from build123d import *

# Parameters (mm, degrees)
SKETCH_1_W             = 180
SKETCH_1_H             = 5
EXTRUDE_1_DEPTH        = 10
SKETCH_2_W             = 3
SKETCH_2_H             = 8
EXTRUDE_2_DEPTH        = 60
SKETCH_5_R             = 2
EXTRUDE_4_DEPTH        = 8
SKETCH_6_W             = 36
SKETCH_6_H             = 4
EXTRUDE_5_DEPTH        = 40
SKETCH_7_W             = 30
SKETCH_7_H             = 5
EXTRUDE_6_DEPTH        = 30
PATTERN_LINEAR_1_COUNT = 2
PATTERN_LINEAR_1_PITCH = 177.5
EXTRUDE_START          = 8
SKETCH_8_R             = 2
EXTRUDE_7_DEPTH        = 8


with BuildPart() as part:
    # 草图1 → 凸台-拉伸1 (new body)
    with BuildSketch(Plane(origin=(0, 0, 0), x_dir=(1, 0, 0), z_dir=(0, 1, 0))):
        Rectangle(SKETCH_1_W, SKETCH_1_H)
    extrude(amount=EXTRUDE_1_DEPTH)

    # 草图2 → 凸台-拉伸2 (add)
    with BuildSketch(Plane(origin=(0, 0, -2.5), x_dir=(-1, 0, 0), z_dir=(0, 0, -1))):
        with Locations((-88.5, 5)):
            Rectangle(SKETCH_2_W, SKETCH_2_H)
    extrude_2 = extrude(amount=EXTRUDE_2_DEPTH)

    # 草图5 → 凸台-拉伸4 (add)
    with BuildSketch(Plane.ZY.offset(-87)):
        with Locations(Location((-59.5, 5, 0), (0, 0, 180))):
            Circle(SKETCH_5_R)
    extrude(amount=EXTRUDE_4_DEPTH)

    # 草图6 → 凸台-拉伸5 (add)
    with BuildSketch(Plane.XY.offset(2.5)):
        with Locations((0, 5)):
            Rectangle(SKETCH_6_W, SKETCH_6_H)
    extrude(amount=EXTRUDE_5_DEPTH)

    # 草图7 → 凸台-拉伸6 (add)
    with BuildSketch(Plane.XZ.offset(-3)):
        with Locations((0, 40)):
            Rectangle(SKETCH_7_W, SKETCH_7_H)
    extrude(amount=EXTRUDE_6_DEPTH)

    # 阵列(线性)1: 凸台-拉伸2 ×2
    with Locations(*[(-i * PATTERN_LINEAR_1_PITCH, 0, 0) for i in range(1, PATTERN_LINEAR_1_COUNT)]):
        add(extrude_2)

    # 草图8 → 凸台-拉伸7 (add)
    with BuildSketch(Plane(origin=(-87.5, 0, 0), x_dir=(0, 0, -1), z_dir=(1, 0, 0)).offset(EXTRUDE_START)):
        with Locations((59.5, 5)):
            Circle(SKETCH_8_R)
    extrude(amount=-EXTRUDE_7_DEPTH)


solid = part.part
Geometry check sheet. Reference: the model listing, model coordinates, mm. A direction names the side the tool comes from. Round coordinates to 2 decimals unless told otherwise and drop trailing zeros. Loops run counter-clockwise (first coordinate to the right, second up) from the corner with the lowest first, then second, coordinate; pieces in that order, holes last.
Item 1: Mould release check, pull along X, two halves, no side actions. Record for faces 4 (the flat face through (79, 5, -59)), 5 (the flat face through (15, -12, 40)), 6 (the flat face through (-1, 0, 0)): pulls with the +X half, pulls with the -X half, needs draft (parallel to the pull), parting line crosses it, or undercut.
Item 2: Cross-section at B-B on y = 5. Record the boundary of the cut face in (x, z).
Item 3: Access from +Z, -Z, +X, -X, +Y, -Y to the whole of each face (thin tool, end or side, straight path). Record for faces 1 (the cylindrical face through (-83.444, 5.601, -61.408)), 2 (the flat face through (0, 7, 22)), 3 (the flat face through (-79.5, 5, -59)).
Item 4: Cross-section at A-A on z = -59.5. Record the boundary of the cut face in (x, y).
Item 5: Cross-section at C-C on x = 67. Record the boundary of the cut face in (y, z).
Item 6: Gauge pin test, flat ends, axial feed: pin 1 (9 mm diameter, centred on x = 2.5, y = -7.5, fed in from -Z); pin 2 (2.5 mm diameter, centred on x = -24, z = 0, fed in from -Y); pin 3 (2.5 mm diameter, centred on x = -88.5, z = -29.5, fed in from +Y). Record the tip position at first contact, or that the pin passes through.
Item 7: Thickness scan on line 1 (X direction, y = 4, z = -45.5); line 2 (Y direction, x = 17, z = 5.5); line 3 (Z direction, x = 7, y = -9.5). Record the ranges inside material, lowest first.
Item 8: Cross-section at D-D on z = 5. Record the boundary of the cut face in (x, y).
Answer sheet:
1. face 4: undercut
1. face 5: pulls with the +X half
1. face 6: needs draft
2. outline: (-90.5, -62.5) - (-87.5, -62.5) - (-87.5, -61.5) - (-79.5, -61.5) - (-79.5, -57.5) - (-87.5, -57.5) - (-87.5, -2.5) - (87, -2.5) - (87, -57.5) - (79, -57.5) - (79, -61.5) - (87, -61.5) - (87, -62.5) - (90, -62.5) - (90, 2.5) - (18, 2.5) - (18, 42.5) - (-18, 42.5) - (-18, 2.5) - (-90, 2.5) - (-90, -2.5) - (-90.5, -2.5) - close
3. face 1: none
3. face 2: +Z, +X, -X, +Y
3. face 3: -Z, +Y, -Y
4. outline: (-90.5, 1) - (-87.5, 1) - (-87.5, 3) - (-79.5, 3) - (-79.5, 7) - (-87.5, 7) - (-87.5, 9) - (-90.5, 9) - close; (79, 3) - (87, 3) - (87, 1) - (90, 1) - (90, 9) - (87, 9) - (87, 7) - (79, 7) - close
5. outline: (0, -2.5) - (10, -2.5) - (10, 2.5) - (0, 2.5) - close
6. pin 1: stops at z = 37.5
6. pin 2: stops at y = 0
6. pin 3: stops at y = 9
7. line 1: x = -90.5 to -87.5, 87 to 90
7. line 2: y = 3 to 7
7. line 3: z = 37.5 to 42.5
8. outline: (-18, 3) - (18, 3) - (18, 7) - (-18, 7) - close
